Check sheet for the modelled part. Datum: model origin and axes. Units: mm. Round coordinates to 2 decimals unless told otherwise and drop trailing zeros. Order: outer loops, then holes, each group sorted by start corner. A loop starts at its lowest first (then second) coordinate and runs counter-clockwise, first axis right, second up. Notation, with made-up numbers: (-6.75, -8.5) -> (1.25, -8.5) arc R24 cw to (1.25, 3.5) -> close; hole circle Ø9 at (30, -9). An arc over 180 degrees is marked (long way). Answer in a Markdown table with one row per item. Add a question column.
1. Material ranges on L1, parallel to Y at x = -55, z = 5.25; L2, parallel to X at y = -8.5, z = 3.5; L3, parallel to X at y = -13, z = 5, recorded low to high. Write a range as from..to.
2. Depth check by flat-ended pin: P1, Ø10, axis at x = 90.5, y = -6, coming from the +Z side. Enter the tip coordinate at first touch or a pass-through.
3. Sectioned sample at C-C, the plane x = -49.5. Record the boundary of the cut face in (y, z).
4. Sectioned sample at A-A, the plane x = 95. Record the boundary of the cut face in (y, z).
5. Sectioned sample at B-B, the plane y = -5. Record the boundary of the cut face in (x, z), then the cut area to 3 significant figures.
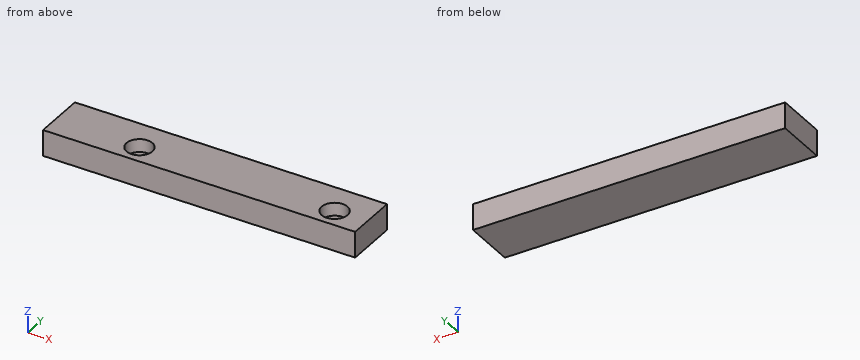
```python
from build123d import *

# Parameters (mm, degrees)
F0_W     = 240
F0_H     = 40
F1_DEPTH = 10
F2_R     = 10
F3_DEPTH = 10


with BuildPart() as f1:
    # F0 (on Top) → F1 (new body, symmetric)
    with BuildSketch(Plane.XY):
        Rectangle(F0_W, F0_H)
    extrude(amount=F1_DEPTH, both=True)

    # F2 (on face) → F3 (cut)
    with BuildSketch(Plane.XY.offset(10)):
        with Locations((-55, -5)):
            Circle(F2_R)
        with Locations((95, -5)):
            Circle(F2_R)
    extrude(amount=-F3_DEPTH, mode=Mode.SUBTRACT)


solid = f1.part
```
Answer key:
| question | item | result |
|---|---|---|
| 1 | L1 | y = -20..-15, 5..20 |
| 1 | L2 | x = -120..-64.37, -45.63..85.63, 104.37..120 |
| 1 | L3 | x = -120..-61, -49..89, 101..120 |
| 2 | P1 | stops at z = 0 |
| 3 | outline | (-20, -10) -> (20, -10) -> (20, 10) -> (3.35, 10) -> (3.35, 0) -> (-13.35, 0) -> (-13.35, 10) -> (-20, 10) -> close |
| 4 | outline | (-20, -10) -> (20, -10) -> (20, 10) -> (5, 10) -> (5, 0) -> (-15, 0) -> (-15, 10) -> (-20, 10) -> close |
| 5 | outline | (-120, -10) -> (120, -10) -> (120, 10) -> (105, 10) -> (105, 0) -> (85, 0) -> (85, 10) -> (-45, 10) -> (-45, 0) -> (-65, 0) -> (-65, 10) -> (-120, 10) -> close |
| 5 | area | 4,400 mm² |
